```python
from build123d import *

# Parameters (mm, degrees)
SKETCH1_W           = 80
SKETCH1_H           = 80
BOSS_EXTRUDE1_DEPTH = 30
SKETCH2_W           = 76
SKETCH2_H           = 76
CUT_EXTRUDE1_DEPTH  = 29
SKETCH3_R           = 2.5
SKETCH3_R_2         = 1.5
BOSS_EXTRUDE5_DEPTH = 20
SKETCH4_R           = 2.5
CUT_EXTRUDE2_DEPTH  = 10
SKETCH5_W           = 26.5
SKETCH5_H           = 15.5
CUT_EXTRUDE3_DEPTH  = 25
SKETCH6_R           = 5.1
CUT_EXTRUDE4_DEPTH  = 10
BOSS_EXTRUDE6_DEPTH = 3
CUT_EXTRUDE5_DEPTH  = 2
SKETCH10_R          = 1
CUT_EXTRUDE6_DEPTH  = 3


with BuildPart() as part:
    # Sketch1 → Boss-Extrude1 (new body)
    with BuildSketch(Plane(origin=(0, 0, 0), x_dir=(1, 0, 0), z_dir=(0, 1, 0))):
        Rectangle(SKETCH1_W, SKETCH1_H)
    extrude(amount=BOSS_EXTRUDE1_DEPTH)

    # Sketch2 → Cut-Extrude1 (cut)
    with BuildSketch(Plane(origin=(0, 30, 0), x_dir=(1, 0, 0), z_dir=(0, 1, 0))):
        Rectangle(SKETCH2_W, SKETCH2_H)
    extrude(amount=-CUT_EXTRUDE1_DEPTH, mode=Mode.SUBTRACT)

    # Sketch3 → Boss-Extrude5 (add)
    with BuildSketch(Plane(origin=(0, 1, 0), x_dir=(1, 0, 0), z_dir=(0, 1, 0))):
        with Locations((-34.5, 34.5)):
            Circle(SKETCH3_R)
        with Locations((-34.5, 34.5)):
            Circle(SKETCH3_R_2, mode=Mode.SUBTRACT)
        with Locations((34.5, 34.5)):
            Circle(SKETCH3_R)
        with Locations((34.5, 34.5)):
            Circle(SKETCH3_R_2, mode=Mode.SUBTRACT)
        with Locations((-34.5, -34.5)):
            Circle(SKETCH3_R)
        with Locations((-34.5, -34.5)):
            Circle(SKETCH3_R_2, mode=Mode.SUBTRACT)
        with Locations((34.5, -34.5)):
            Circle(SKETCH3_R)
        with Locations((34.5, -34.5)):
            Circle(SKETCH3_R_2, mode=Mode.SUBTRACT)
    extrude(amount=BOSS_EXTRUDE5_DEPTH)

    # Sketch4 → Cut-Extrude2 (cut)
    with BuildSketch(Plane.XZ):
        with Locations((-20, -18)):
            Circle(SKETCH4_R)
    extrude(amount=-CUT_EXTRUDE2_DEPTH, mode=Mode.SUBTRACT)

    # Sketch5 → Cut-Extrude3 (cut)
    with BuildSketch(Plane.XZ):
        with Locations((11.75, 22.941412849)):
            Rectangle(SKETCH5_W, SKETCH5_H)
    extrude(amount=-CUT_EXTRUDE3_DEPTH, mode=Mode.SUBTRACT)

    # Sketch6 → Cut-Extrude4 (cut)
    with BuildSketch(Plane.XY.offset(40)):
        with Locations((-20, 15.536781198)):
            Circle(SKETCH6_R)
    extrude(amount=-CUT_EXTRUDE4_DEPTH, mode=Mode.SUBTRACT)

    # Sketch11 → Boss-Extrude6 (add)
    with BuildSketch(Plane(origin=(0, 1, 0), x_dir=(1, 0, 0), z_dir=(0, 1, 0))):
        with BuildLine():
            Line((-3.6, -5.131412849), (-3.6, -13.131412849))
            ThreePointArc((-3.6, -13.131412849), (2.056854249, -10.788267099), (4.4, -5.131412849))
            Line((4.4, -5.131412849), (-3.6, -5.131412849))
        make_face()
        with BuildLine():
            Line((19.1, -5.131412849), (27.1, -5.131412849))
            Line((27.1, -5.131412849), (27.1, -13.131412849))
            ThreePointArc((27.1, -13.131412849), (21.443145751, -10.788267099), (19.1, -5.131412849))
        make_face()
        with BuildLine():
            Line((27.1, -28.491412849), (27.1, -36.491412849))
            Line((27.1, -36.491412849), (19.1, -36.491412849))
            ThreePointArc((19.1, -36.491412849), (21.443145751, -30.8345586), (27.1, -28.491412849))
        make_face()
        with BuildLine():
            Line((4.4, -36.491412849), (-3.6, -36.491412849))
            Line((-3.6, -36.491412849), (-3.6, -28.491412849))
            ThreePointArc((-3.6, -28.491412849), (2.056854249, -30.8345586), (4.4, -36.491412849))
        make_face()
    extrude(amount=BOSS_EXTRUDE6_DEPTH)

    # Sketch12 → Cut-Extrude5 (cut)
    with BuildSketch(Plane(origin=(0, 1, 0), x_dir=(1, 0, 0), z_dir=(0, 1, 0))):
        with BuildLine():
            Line((-2.9, -13.100729005), (-2.9, -5.831412849))
            Line((-2.9, -5.831412849), (4.369316156, -5.831412849))
            ThreePointArc((4.369316156, -5.831412849), (2.240182749, -10.971595598), (-2.9, -13.100729005))
        make_face()
        with BuildLine():
            Line((19.130683844, -5.831412849), (26.4, -5.831412849))
            Line((26.4, -5.831412849), (26.4, -13.100729005))
            ThreePointArc((26.4, -13.100729005), (21.259817251, -10.971595598), (19.130683844, -5.831412849))
        make_face()
        with BuildLine():
            Line((26.4, -35.491412849), (26.4, -28.522096693))
            ThreePointArc((26.4, -28.522096693), (21.471949286, -30.563362135), (19.430683844, -35.491412849))
            Line((19.430683844, -35.491412849), (26.4, -35.491412849))
        make_face()
        with BuildLine():
            Line((4.337253933, -35.491412849), (-2.9, -35.491412849))
            Line((-2.9, -35.491412849), (-2.9, -28.254158916))
            ThreePointArc((-2.9, -28.254158916), (2.217511333, -30.373901516), (4.337253933, -35.491412849))
        make_face()
    extrude(amount=CUT_EXTRUDE5_DEPTH, mode=Mode.SUBTRACT)

    # Sketch10 → Cut-Extrude6 (cut)
    with BuildSketch(Plane(origin=(0, 1, 0), x_dir=(1, 0, 0), z_dir=(0, 1, 0))):
        with Locations((0.2, -8.931412849)):
            Circle(SKETCH10_R)
        with Locations((23.3, -8.931412849)):
            Circle(SKETCH10_R)
        with Locations((0.2, -33.191412849)):
            Circle(SKETCH10_R)
        with Locations((23.3, -33.191412849)):
            Circle(SKETCH10_R)
    extrude(amount=CUT_EXTRUDE6_DEPTH, mode=Mode.SUBTRACT)


solid = part.part
```
Geometry: final body of the model. Coordinates: model frame, mm. A direction names the side the tool comes from. Round coordinates to 2 decimals unless told otherwise and drop trailing zeros. Write each loop counter-clockwise with the first axis right and the second up, starting at its lowest first coordinate (ties: lowest second). Pieces come first, ordered by that corner, then holes.
Item 1: Section query D-D (x = 6). Return loops of the section in (y, z), plus the area to 4 significant figures.
Item 2: Mould query, pull axis Z, two halves, no side actions, for faces 1 (the face through (-1, 15, -40)), 2 (the face through (27.1, 2, 9)), 3 (the face through (-20.664, 20.593, 39.014)). Classes: +Z half, -Z half, draft (parallel to the pull), parting line (faces both ways), or undercut.
Item 3: Section query A-A (y = 6.25). Give the number of separate pieces and of enclosed holes in the cut face, plus the area to 3 significant figures.
Item 4: Pin query (flat end, axial travel): P1, Ø2.5, axis at x = 1.5, z = 30.5, coming from the +Y side; P2, Ø1.5, axis at x = -35, z = 35, coming from the +Y side. Return the tip coordinate at first contact, or that it passes through.
Item 5: Material intervals for L1, parallel to Z at x = 34.5, y = 11; L2, parallel to X at y = 18, z = -16, sorted ascending.
Item 6: Section query C-C (x = -20). Return loops of the section in (y, z).
Item 7: Set-up query: faces 4 (the face through (1, 2, 5.831)), 5 (the face through (36, 21, 36)), 6 (the face through (40, 15, 1)). Return all of +Z, -Z, +X, -X, +Y, -Y with unobstructed straight access to the full face (end or side cutting, diameter ignored); none if empty.
Item 8: Section query B-B (z = -18). Return loops of the section in (x, y).
Completed:
1. outline: (0, -40) - (30, -40) - (30, -38) - (1, -38) - (1, 15.19) - (0, 15.19) - close; (0, 30.69) - (1, 30.69) - (1, 38) - (30, 38) - (30, 40) - (0, 40) - close
1. area: 180.5 mm2
2. face 1: -Z half
2. face 2: undercut
2. face 3: draft
3. separate pieces: 5
3. enclosed holes: 5
3. area: 674 mm2
4. P1: stops at y = 4
4. P2: stops at y = 1
5. L1: z = -40 to -38, -37 to -36, -33 to -32, 32 to 33, 36 to 37, 38 to 40
5. L2: x = -40 to -38, 38 to 40
6. outline: (0, -40) - (30, -40) - (30, -38) - (1, -38) - (1, -20.5) - (0, -20.5) - close; (0, -15.5) - (1, -15.5) - (1, 38) - (10.44, 38) - (10.44, 40) - (0, 40) - close; (20.64, 38) - (30, 38) - (30, 40) - (20.64, 40) - close
7. face 4: none
7. face 5: +Y
7. face 6: +Z, -Z, +X, +Y, -Y
8. outline: (-40, 0) - (-22.5, 0) - (-22.5, 1) - (-38, 1) - (-38, 30) - (-40, 30) - close; (-17.5, 0) - (40, 0) - (40, 30) - (38, 30) - (38, 1) - (-17.5, 1) - close
